Work out the finished part from the listing and answer in its coordinate system (mm). A direction names the side the tool comes from. Coordinates: 2 decimals unless noted, no trailing zeros. Write each loop counter-clockwise with the first axis right and the second up, starting at its lowest first coordinate (ties: lowest second). Pieces come first, ordered by that corner, then holes. Notation, with made-up numbers: (70.5, 72) - (96.5, 72) arc R30 ccw to (96.5, 99) - close; hole circle Ø6 at (-22, 16.25). An arc over 180 degrees is marked (long way). Answer as a JSON object with one key per item and string values. Group by question number.
from build123d import *

# Parameters (mm, degrees)
PAD_DEPTH       = 3
SKETCH002_W     = 20
SKETCH002_H     = 20
PAD001_DEPTH    = 20
FILLET_R        = 5
SKETCH003_R     = 1.9
POCKET_DEPTH    = 125.001
SKETCH004_R     = 7
POCKET001_DEPTH = 23.001
SKETCH005_R     = 1.6
POCKET002_DEPTH = 3.001


with BuildPart() as part:
    # Sketch → Pad (new body)
    with BuildSketch(Plane.XY):
        with BuildLine():
            Line((-80, 65), (80, 65))
            ThreePointArc((85, 60), (83.535534, 63.535534), (80, 65))
            Line((85, 60), (85, -60))
            ThreePointArc((80, -65), (83.535534, -63.535534), (85, -60))
            Line((80, -65), (-80, -65))
            ThreePointArc((-85, -60), (-83.535534, -63.535534), (-80, -65))
            Line((-85, -60), (-85, 60))
            ThreePointArc((-80, 65), (-83.535534, 63.535534), (-85, 60))
        make_face()
    extrude(amount=PAD_DEPTH)

    # Sketch002 → Pad001 (new body)
    with BuildSketch(Plane.XY.offset(3)):
        with Locations((-70, 50)):
            Rectangle(SKETCH002_W, SKETCH002_H)
        with Locations((70, 50)):
            Rectangle(SKETCH002_W, SKETCH002_H)
        with Locations((70, -50)):
            Rectangle(SKETCH002_W, SKETCH002_H)
        with Locations((-70, -50)):
            Rectangle(SKETCH002_W, SKETCH002_H)
    extrude(amount=PAD001_DEPTH)

    # Fillet
    fillet_edges = [part.edges().sort_by_distance(p)[0] for p in [
        (-80, 60, 13),
        (80, 60, 13),
        (-80, -60, 13),
        (80, -60, 13),
    ]]
    fillet(fillet_edges, radius=FILLET_R)

    # Sketch003 → Pocket (cut, through all)
    with BuildSketch(Plane.XZ.offset(60)):
        with Locations((-70, 14)):
            Circle(SKETCH003_R)
        with Locations((70, 14)):
            Circle(SKETCH003_R)
    extrude(amount=-POCKET_DEPTH, mode=Mode.SUBTRACT)

    # Sketch004 → Pocket001 (cut, through all)
    with BuildSketch(Plane.XY.offset(23)):
        with Locations((-69.859705, 49.927501)):
            Circle(SKETCH004_R)
        with Locations((69.859705, 49.927501)):
            Circle(SKETCH004_R)
        with Locations((69.859705, -49.927501)):
            Circle(SKETCH004_R)
        with Locations((-69.859705, -49.927501)):
            Circle(SKETCH004_R)
    extrude(amount=-POCKET001_DEPTH, mode=Mode.SUBTRACT)

    # Sketch005 → Pocket002 (cut, through all)
    with BuildSketch(Plane.XY.offset(3)):
        with Locations((-54.025897, -39.472939)):
            Circle(SKETCH005_R)
        with Locations((-46.525897, -39.472939)):
            Circle(SKETCH005_R)
        with Locations((-39.025897, -39.472939)):
            Circle(SKETCH005_R)
    extrude(amount=-POCKET002_DEPTH, mode=Mode.SUBTRACT)


solid = part.part
Q1. For a pull along X with two mould halves and no side action, classify faces 5 (the face through (-84, -63, 1)), 6 (the face through (-60, -50, 13)), 7 (the face through (71.812, 58.288, 14.571)), 8 (the face through (1, 1, 0)) as +X half, -X half, draft (parallel to the pull), parting line (faces both ways), or undercut.
Q2. Section A-A on z = 8.25 is taken. Determine the outline of the cut face in (x, y), plus the area to 3 significant figures.
Q3. Consider L1, parallel to X at y = 40.8, z = 14; L2, parallel to X at y = 58.5, z = 14.5; L3, parallel to Z at x = 70, y = -42.15. Determine where each line is inside the solid, lowest interval first. Write a range as from..to.
Q4. Flat-ended cylindrical pins translate along their axes: pin 1 Ø3 at (x, z) = (70, 14) entering from +Y; pin 2 Ø10 at (y, z) = (-50, 9) entering from +X; pin 3 Ø4.5 at (x, z) = (-65, 16) entering from -Y; pin 4 Ø12 at (x, y) = (-64.5, -21) entering from +Z. Find the tip coordinate at first contact, or state that the pin passes through.
Q5. A tool of negligible diameter and unlimited length cuts with its end or side. For faces 1 (the face through (70, -40, 11)), 2 (the face through (67, 60, 13)), 3 (the face through (-80, -48, 13)), 4 (the face through (-68, -60, 13)), from which of +Z, -Z, +X, -X, +Y, -Y can it reach the whole face along a straight path? Write none if from no direction.
Q6. Section B-B on y = -48 is taken. Determine the outline of the cut face in (x, z).
Q7. Section D-D on y = -31 is taken. Determine the outline of the cut face in (x, z).
Q8. Section C-C on x = 43.5 is taken. Determine the outline of the cut face in (y, z).
Numbers:
{
 "1": {"face 5": "-X half", "face 6": "undercut", "face 7": "undercut", "face 8": "draft"},
 "2": {"outline": "(-80, -55) arc R5 ccw to (-75, -60) - (-60, -60) - (-60, -40) - (-80, -40) - close; (-80, 40) - (-60, 40) - (-60, 60) - (-75, 60) arc R5 ccw to (-80, 55) - close; (60, -60) - (75, -60) arc R5 ccw to (80, -55) - (80, -40) - (60, -40) - close; (60, 40) - (80, 40) - (80, 55) arc R5 ccw to (75, 60) - (60, 60) - close; hole circle Ø14 at (-69.86, -49.93); hole circle Ø14 at (-69.86, 49.93); hole circle Ø14 at (69.86, -49.93); hole circle Ø14 at (69.86, 49.93)", "area": "963 mm²"},
 "3": {"L1": "x = -80..-71.9, -68.1..-60, 60..68.1, 71.9..80", "L2": "x = -78.57..-71.83, -68.17..-60, 60..68.17, 71.83..78.57", "L3": "z = 0..12.1, 15.9..23"},
 "4": {"pin 1": "passes through", "pin 2": "stops at x = 80", "pin 3": "stops at y = -60", "pin 4": "stops at z = 3"},
 "5": {"face 1": "+Z, +X, -X", "face 2": "+Z, +X, -X, +Y", "face 3": "+Z, -X, +Y, -Y", "face 4": "+Z, +X, -X, -Y"},
 "6": {"outline": "(-85, 0) - (-76.59, 0) - (-76.59, 23) - (-80, 23) - (-80, 3) - (-85, 3) - close; (-63.13, 0) - (63.13, 0) - (63.13, 23) - (60, 23) - (60, 3) - (-60, 3) - (-60, 23) - (-63.13, 23) - close; (76.59, 0) - (85, 0) - (85, 3) - (80, 3) - (80, 23) - (76.59, 23) - close"},
 "7": {"outline": "(-85, 0) - (85, 0) - (85, 3) - (-85, 3) - close"},
 "8": {"outline": "(-65, 0) - (65, 0) - (65, 3) - (-65, 3) - close"}
}
